```python
from build123d import *

# Parameters (mm, degrees)
BASES_R        = 4.8
BASE_DEPTH     = 3.2
FLANGES_R      = 6.5
FLANGE_DEPTH   = 1
TOPBORES_R     = 4
TOPBORE_DEPTH  = 4
THRUHOLES_R    = 2
THRUHOLE_DEPTH = 5.4


with BuildPart() as part:
    # BaseS → Base (new body, symmetric)
    with BuildSketch(Plane(origin=(0, 0, 0), x_dir=(1, 0, 0), z_dir=(0, 1, 0))):
        Circle(BASES_R)
    extrude(amount=BASE_DEPTH, both=True)

    # FlangeS → Flange (add)
    with BuildSketch(Plane(origin=(0, 3.2, 0), x_dir=(1, 0, 0), z_dir=(0, 1, 0))):
        Circle(FLANGES_R)
    flange = extrude(amount=FLANGE_DEPTH)

    # TopBoreS → TopBore (cut)
    with BuildSketch(Plane(origin=(0, 4.2, 0), x_dir=(1, 0, 0), z_dir=(0, 1, 0))):
        Circle(TOPBORES_R)
    topbore = extrude(amount=-TOPBORE_DEPTH, mode=Mode.SUBTRACT)

    # BoreVM: Flange, TopBore across plane
    add(flange.mirror(Plane.ZX))
    add(topbore.mirror(Plane.ZX), mode=Mode.SUBTRACT)

    # ThruHoleS → ThruHole (cut, through all)
    with BuildSketch(Plane(origin=(0, 0.2, 0), x_dir=(1, 0, 0), z_dir=(0, 1, 0))):
        Circle(THRUHOLES_R)
    extrude(amount=-THRUHOLE_DEPTH, mode=Mode.SUBTRACT)


solid = part.part
```
Build history of the part. All positions in model axes, mm. A direction names the side the tool comes from. Give positions to 0.01 mm unless a question says otherwise; leave off trailing zeros. Order: outer loops, then holes, each group sorted by start corner. A loop starts at its lowest first (then second) coordinate and runs counter-clockwise, first axis right, second up. Notation, with made-up numbers: M 32.25,-15 L 71.25,-15 A11 ccw 71.25,0 Z; hole C -26,68.25 d3. An arc over 180 degrees is marked long. Return JSON: item names as keys, results as strings.
Q1. Band-saw the part on B-B (z = 0). Give the cut face in (x, y), then the cut area to 3 significant figures.
Answer list:
{"outline": "M -6.5,-4.2 L -4,-4.2 L -4,-0.2 L -2,-0.2 L -2,0.2 L -4,0.2 L -4,4.2 L -6.5,4.2 L -6.5,3.2 L -4.8,3.2 L -4.8,-3.2 L -6.5,-3.2 Z; M 2,-0.2 L 4,-0.2 L 4,-4.2 L 6.5,-4.2 L 6.5,-3.2 L 4.8,-3.2 L 4.8,3.2 L 6.5,3.2 L 6.5,4.2 L 4,4.2 L 4,0.2 L 2,0.2 Z", "area": "21.8 mm^2"}
Q2. Wall check: probe 1 along Y at (x, z) = (-0.5, 5); probe 2 along X at (y, z) = (0, 0); probe 3 along X at (y, z) = (3.3, 0). Give the ranges that are in metal, low to high. Write a range as from..to.
Answer list:
{"probe 1": "y = -4.2..-3.2, 3.2..4.2", "probe 2": "x = -4.8..-2, 2..4.8", "probe 3": "x = -6.5..-4, 4..6.5"}
Q3. Band-saw the part on D-D (z = -4.5). Give the cut face in (x, y), then the cut area to 3 significant figures.
Answer list:
{"outline": "M -4.69,-4.2 L 4.69,-4.2 L 4.69,-3.2 L 1.67,-3.2 L 1.67,3.2 L 4.69,3.2 L 4.69,4.2 L -4.69,4.2 L -4.69,3.2 L -1.67,3.2 L -1.67,-3.2 L -4.69,-3.2 Z", "area": "40.1 mm^2"}
Q4. Flat gauge pins, fed straight in: pin 1 (3 mm diameter, centred on y = 1, z = -5, fed in from -X); pin 2 (1.5 mm diameter, centred on x = 1.5, z = 2, fed in from +Y); pin 3 (4 mm diameter, centred on x = 4.5, y = 0, fed in from -Z). Where does each tip first touch, or does it go through?
Answer list:
{"pin 1": "stops at x = -3.28", "pin 2": "stops at y = 0.2", "pin 3": "stops at z = -4.1"}
Q5. 3-axis set-ups, long thin cutter, end or side, ignore diameter. For faces 1 (the face through (-1, -3.2, 5)), 2 (the face through (0, 0, 2)), 3 (the face through (3, 4.2, -3)), 4 (the face through (-2, -0.2, 1)), 5 (the face through (-2, 0.2, 1)): which of +Z, -Z, +X, -X, +Y, -Y reach the whole face in a straight line?
Answer list:
{"face 1": "none", "face 2": "+Y, -Y", "face 3": "+Z, -Z, +X, -X, +Y", "face 4": "-Y", "face 5": "+Y"}
Q6. Band-saw the part on A-A (x = 0). Give the cut face in (y, z).
Answer list:
{"outline": "M -4.2,-6.5 L -3.2,-6.5 L -3.2,-4.8 L 3.2,-4.8 L 3.2,-6.5 L 4.2,-6.5 L 4.2,-4 L 0.2,-4 L 0.2,-2 L -0.2,-2 L -0.2,-4 L -4.2,-4 Z; M -4.2,4 L -0.2,4 L -0.2,2 L 0.2,2 L 0.2,4 L 4.2,4 L 4.2,6.5 L 3.2,6.5 L 3.2,4.8 L -3.2,4.8 L -3.2,6.5 L -4.2,6.5 Z"}
Q7. Two-plate mould, pull along Z, no slides. Class faces 6 (the face through (-5.158, -3.693, 3.955)), 7 (the face through (-0.867, -2.228, 3.905)), 8 (the face through (-1, 3.2, 5)): pulls with the +Z half, pulls with the -Z half, needs draft (parallel to the pull), parting line crosses it, or undercut.
Answer list:
{"face 6": "parting line crosses it", "face 7": "undercut", "face 8": "needs draft"}
Q8. Band-saw the part on C-C (x = -2.5). Give the cut face in (y, z).
Answer list:
{"outline": "M -4.2,-6 L -3.2,-6 L -3.2,-4.1 L 3.2,-4.1 L 3.2,-6 L 4.2,-6 L 4.2,-3.12 L 0.2,-3.12 L 0.2,3.12 L 4.2,3.12 L 4.2,6 L 3.2,6 L 3.2,4.1 L -3.2,4.1 L -3.2,6 L -4.2,6 L -4.2,3.12 L -0.2,3.12 L -0.2,-3.12 L -4.2,-3.12 Z"}
